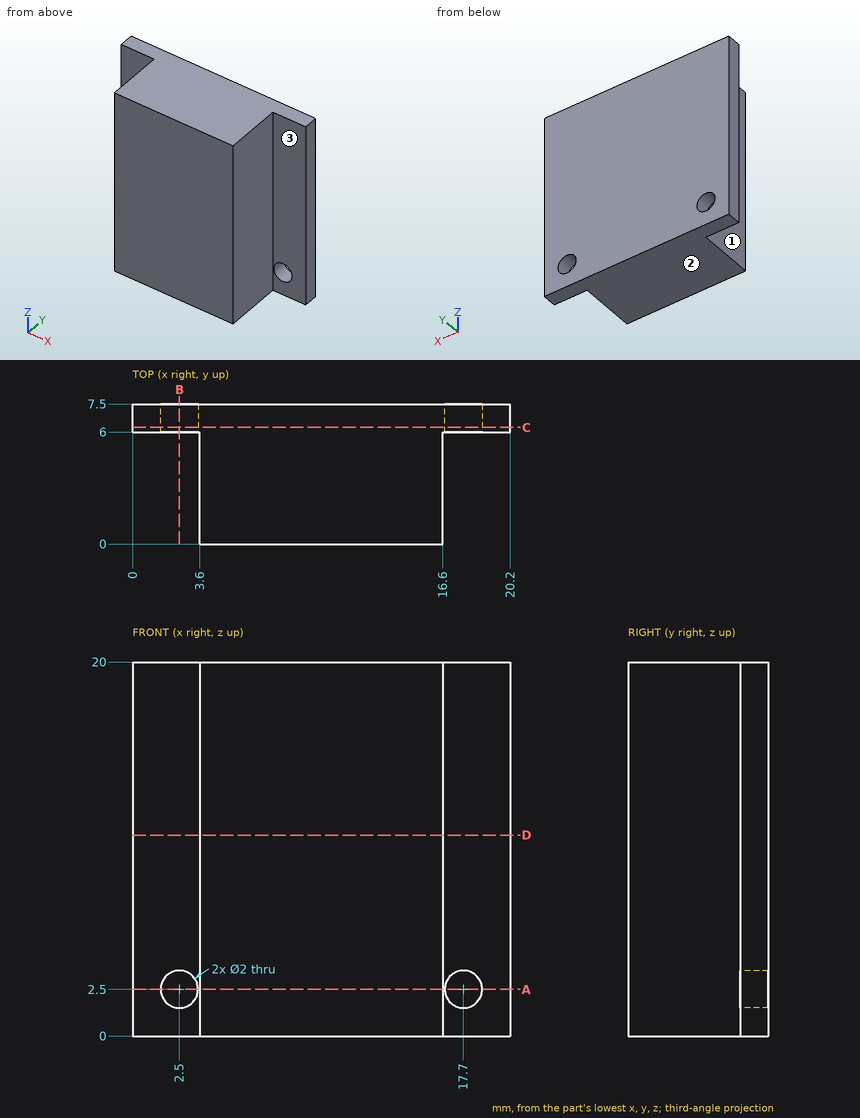
Job drawing, mm, ordinate dimensions from the low corner. One solid piece. A direction names the side the tool comes from. Round coordinates to 2 decimals unless told otherwise and drop trailing zeros. Write each loop counter-clockwise with the first axis right and the second up, starting at its lowest first coordinate (ties: lowest second). Pieces come first, ordered by that corner, then holes.
1) 3-axis set-ups, long thin cutter, end or side, ignore diameter. For the marked faces 1, 2 and 3: which of +Z, -Z, +X, -X, +Y, -Y reach the whole face in a straight line?
2) Band-saw the part on A-A, the plane z = 2.5. List the corners of the cut face in (x, y).
3) Band-saw the part on D-D, the plane z = 10.75. List the corners of the cut face in (x, y), and give its area (3 significant figures).
4) Drill centre lines: probe 1 along X at (y, z) = (6.7, 2.5); probe 2 along Z at (x, y) = (17.7, 6.85); probe 3 along Y at (x, z) = (18, 13.25). Where is each one in solid material? Low to high.
5) Band-saw the part on B-B, the plane x = 2.5. List the corners of the cut face in (y, z).
6) Pin check, flat tips, straight feed: pin 1 (5 mm diameter, centred on x = 4.5, z = 5, fed in from -Y); pin 2 (1.8 mm diameter, centred on y = 3.5, z = 6.5, fed in from -X); pin 3 (3 mm diameter, centred on x = 19, z = 9.5, fed in from -Y). Stop position of each tip, or through.
7) Band-saw the part on C-C, the plane y = 6.25. List the corners of the cut face in (x, z), and give its area (3 significant figures).
Ans:
1. face 1: +Z, -Z, -X, -Y
1. face 2: -Z, +X, -X, +Y, -Y
1. face 3: +Z, -Z, +X, -Y
2. outline: (0, 6) - (1.5, 6) - (1.5, 7.5) - (0, 7.5) - close; (3.5, 6) - (3.6, 6) - (3.6, 0) - (16.6, 0) - (16.6, 6) - (16.7, 6) - (16.7, 7.5) - (3.5, 7.5) - close; (18.7, 6) - (20.2, 6) - (20.2, 7.5) - (18.7, 7.5) - close
3. outline: (0, 6) - (3.6, 6) - (3.6, 0) - (16.6, 0) - (16.6, 6) - (20.2, 6) - (20.2, 7.5) - (0, 7.5) - close
3. area: 108 mm2
4. probe 1: x = 0 to 1.5, 3.5 to 16.7, 18.7 to 20.2
4. probe 2: z = 0 to 1.5, 3.5 to 20
4. probe 3: y = 6 to 7.5
5. outline: (6, 0) - (7.5, 0) - (7.5, 1.5) - (6, 1.5) - close; (6, 3.5) - (7.5, 3.5) - (7.5, 20) - (6, 20) - close
6. pin 1: stops at y = 0
6. pin 2: stops at x = 3.6
6. pin 3: stops at y = 6
7. outline: (0, 0) - (20.2, 0) - (20.2, 20) - (0, 20) - close; hole circle Ø2 at (2.5, 2.5); hole circle Ø2 at (17.7, 2.5)
7. area: 398 mm2
